```python
from build123d import *

# Parameters (mm, degrees)
F0_R     = 10
F1_DEPTH = 10
F3_DEPTH = 25


with BuildPart() as f1:
    # F0 (on Front) → F1 (new body)
    with BuildSketch(Plane.XZ):
        with BuildLine():
            Line((96.709934, 115.595525), (-43.290066, 115.595525))
            ThreePointArc((-43.290066, 115.595525), (-46.8256, 114.131058), (-48.290066, 110.595525))
            Line((-48.290066, 110.595525), (-48.290066, -53.404475))
            ThreePointArc((-48.290066, -53.404475), (-46.8256, -56.940009), (-43.290066, -58.404475))
            Line((-43.290066, -58.404475), (96.709934, -58.404475))
            ThreePointArc((96.709934, -58.404475), (100.245467, -56.940009), (101.709934, -53.404475))
            Line((101.709934, -53.404475), (101.709934, 110.595525))
            ThreePointArc((101.709934, 110.595525), (100.245467, 114.131058), (96.709934, 115.595525))
        make_face()
        with Locations((-13.290066, -23.404475)):
            Circle(F0_R, mode=Mode.SUBTRACT)
        with Locations((66.709934, -23.404475)):
            Circle(F0_R, mode=Mode.SUBTRACT)
        with Locations((-13.290066, 80.595525)):
            Circle(F0_R, mode=Mode.SUBTRACT)
        with Locations((66.709934, 80.595525)):
            Circle(F0_R, mode=Mode.SUBTRACT)
    extrude(amount=F1_DEPTH)

    # F2 (on face) → F3 (cut)
    with BuildSketch(Plane.XZ.offset(10)):
        with BuildLine():
            Line((128.527537, 115.595525), (16.709934, 115.595525))
            Line((16.709934, 115.595525), (16.709934, 95.595525))
            ThreePointArc((16.709934, 95.595525), (15.245467, 92.059991), (11.709934, 90.595525))
            Line((11.709934, 90.595525), (-13.290066, 90.595525))
            ThreePointArc((-13.290066, 90.595525), (-23.288771, 80.756455), (-13.611886, 70.600704))
            Line((-13.611886, 70.600704), (11.709934, 70.600704))
            ThreePointArc((11.709934, 70.600704), (15.245467, 69.136238), (16.709934, 65.600704))
            Line((16.709934, 65.600704), (16.709934, -8.404598))
            ThreePointArc((16.709934, -8.404598), (15.245467, -11.940131), (11.709934, -13.404598))
            Line((11.709934, -13.404598), (-13.339475, -13.404598))
            ThreePointArc((-13.339475, -13.404598), (-23.48642, -23.329165), (-13.48718, -33.402533))
            Line((-13.48718, -33.402533), (11.709934, -33.402533))
            ThreePointArc((11.709934, -33.402533), (15.245467, -34.866999), (16.709934, -38.402533))
            Line((16.709934, -38.402533), (16.709934, -58.404475))
            Line((16.709934, -58.404475), (128.527537, -58.404475))
            Line((128.527537, -58.404475), (128.527537, 115.595525))
        make_face()
    extrude(amount=-F3_DEPTH, mode=Mode.SUBTRACT)


solid = f1.part
```
Model file for the job. Use its own axes, mm. A direction names the side the tool comes from. Coordinates: 2 decimals unless noted, no trailing zeros. Write each loop counter-clockwise with the first axis right and the second up, starting at its lowest first coordinate (ties: lowest second). Pieces come first, ordered by that corner, then holes. Notation, with made-up numbers: (-31.5, -11) - (-21.5, -11) arc R32 cw to (-21.5, 22) - close; hole circle Ø3 at (26.5, -38). An arc over 180 degrees is marked (long way). One line per item, written item: value. Start each with the question number.
1. Probe line 1 (Z direction, x = -4, y = -3.5); line 2 (Z direction, x = 12.5, y = -3.75); line 3 (X direction, y = -8, z = 76). List the from-to ranges inside material, lowest first. Write a range as from..to.
2. Slice it at A-A (x = 3). Write the cut outline in (y, z), plus the area to 3 significant figures.
3. Flat gauge pin, fed straight in: pin 1 (3 mm diameter, centred on y = -4, z = -16.5, fed in from +X). Where does the tip first touch, or does it go through?
4. Mould opens along Z. For faces 3 (the flat face through (-13, -5, 115.596)), 4 (the flat face through (16.71, -5, 106)), 5 (the flat face through (-1, -5, -33.403)) say: released by +Z, released by -Z, zero draft, split by the parting line, or undercut.
5. Tool access for faces 1 (the flat face through (-16, 0, 30)), 2 (the cylindrical face through (15.284, -5.07, -11.901)): list every direction of +Z, -Z, +X, -X, +Y, -Y with a clear straight run to the whole face (end or side of a thin tool).
6. Slice it at D-D (z = 87.5). Write the cut outline in (x, y), plus the area to 3 significant figures.
7. Slice it at C-C (z = -31.5). Write the cut outline in (x, y), plus the area to 3 significant figures.
Answers below:
1. line 1: z = -58.4..-33.4, -13.4..70.6, 90.6..115.6
1. line 2: z = -58.4..-33.47, -13.34..70.54, 90.66..115.6
1. line 3: x = -48.29..-22.17
2. outline: (-10, -58.4) - (0, -58.4) - (0, -33.4) - (-10, -33.4) - close; (-10, -13.4) - (0, -13.4) - (0, 70.6) - (-10, 70.6) - close; (-10, 90.6) - (0, 90.6) - (0, 115.6) - (-10, 115.6) - close
2. area: 1,340 mm^2
3. pin 1: stops at x = -18.91
4. face 3: released by +Z
4. face 4: zero draft
4. face 5: undercut
5. face 1: +Z, -Z, +X, -X, +Y
5. face 2: +X, +Y, -Y
6. outline: (-48.29, -10) - (-20.52, -10) - (-20.52, 0) - (-48.29, 0) - close
6. area: 278 mm^2
7. outline: (-48.29, -10) - (-19.35, -10) - (-19.35, 0) - (-48.29, 0) - close
7. area: 289 mm^2
